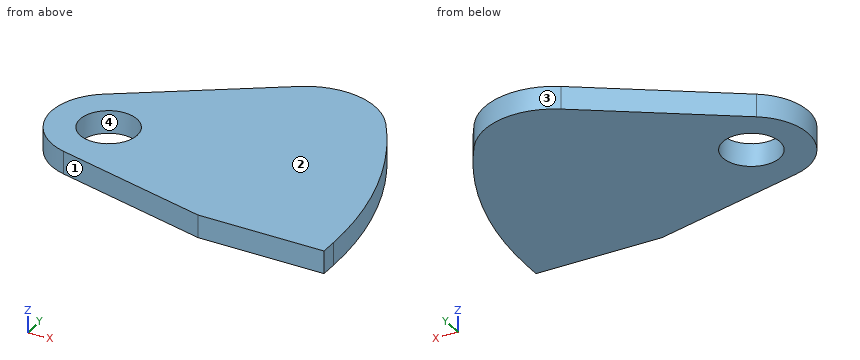
from build123d import *

# Parameters (mm, degrees)
SKETCH_1_R      = 5
EXTRUDE_1_DEPTH = 4


with BuildPart() as part:
    # Эскиз1 → Бобышка-Вытянуть1 (new body)
    with BuildSketch(Plane.XY):
        with BuildLine():
            Line((10.65, 0), (10.65, -3))
            Line((10.65, -3), (-11.397789553, -3))
            Line((-11.397789553, -3), (-38.677904755, 3.651503117))
            ThreePointArc((-38.677904755, 3.651503117), (-46.153775079, 11.6113462), (-41.890065439, 21.664630197))
            Line((-41.890065439, 21.664630197), (-17.065107401, 38.361673869))
            ThreePointArc((-17.065107401, 38.361673869), (-7.827814909, 40.223299164), (0.014835138, 34.999692982))
            ThreePointArc((0.014835138, 34.999692982), (7.932514626, 18.289923732), (10.65, 0))
        make_face()
        with Locations((-36.309076923, 13.366885492)):
            Circle(SKETCH_1_R, mode=Mode.SUBTRACT)
    extrude(amount=EXTRUDE_1_DEPTH)


solid = part.part
Read the model definition and answer for the solid it produces. Units are mm, in the model's axes. Face numbers are marked on the shaded views. Coordinates: 2 decimals unless noted, no trailing zeros. Order: outer loops, then holes, each group sorted by start corner. A loop starts at its lowest first (then second) coordinate and runs counter-clockwise, first axis right, second up. Notation, with made-up numbers: (41.25, 30.5) -> (47.25, 30.5) arc R22 cw to (47.25, 47.5) -> close; hole circle Ø2 at (82.25, -24.5). An arc over 180 degrees is marked (long way). Answer as a JSON object with one key per item and string values.
1) A cutting plane is placed at A-A, the plane y = 17.5. Determine the outline of the cut face in (x, z), plus the area to 3 significant figures.
Model answer:
{"outline": "(-45.41, 0) -> (-39.12, 0) -> (-39.12, 4) -> (-45.41, 4) -> close; (-33.5, 0) -> (8.17, 0) -> (8.17, 4) -> (-33.5, 4) -> close", "area": "192 mm²"}
2) A cutting plane is placed at B-B, the plane z = 1.7. Determine the outline of the cut face in (x, y).
Model answer:
{"outline": "(-41.89, 21.66) arc R10 ccw to (-38.68, 3.65) -> (-11.4, -3) -> (10.65, -3) -> (10.65, 0) arc R62.91 ccw to (0.01, 35) arc R12.3 ccw to (-17.07, 38.36) -> close; hole circle Ø10 at (-36.31, 13.37)"}
3) Each of these flat-tipped pins is pushed along its axis until it touches: pin 1 (1 mm diameter, centred on y = 27, z = 3, fed in from -X); pin 2 (8 mm diameter, centred on x = -23.5, y = 16, fed in from -Z); pin 3 (1 mm diameter, centred on x = -34.5, z = 3.5, fed in from +Y); pin 4 (1.5 mm diameter, centred on y = 9, z = 2, fed in from +X). Where does it stop, or does it pass through?
Model answer:
{"pin 1": "stops at x = -34.7", "pin 2": "stops at z = 0", "pin 3": "stops at y = 26.97", "pin 4": "stops at x = 10.11"}
4) The mould has two halves that part along X. Classify the marked faces 1, 2, 3 and 4: released by +X, released by -X, zero draft, split by the parting line, or undercut.
Model answer:
{"face 1": "released by -X", "face 2": "zero draft", "face 3": "split by the parting line", "face 4": "undercut"}
5) Consider line 1 along Y through (x, z) = (-35.5, 0.35); line 2 along X through (y, z) = (9.5, 1.4); line 3 along X through (y, z) = (15.5, 2.4). Determine where each line is inside the solid, lowest interval first. Write a range as from..to.
Model answer:
{"line 1": "y = 2.88..8.43, 18.3..25.96", "line 2": "x = -45.53..-39.48, -33.14..9.93", "line 3": "x = -46.08..-40.83, -31.79..8.71"}
6) A cutting plane is placed at D-D, the plane y = 25.5. Determine the outline of the cut face in (x, z).
Model answer:
{"outline": "(-36.19, 0) -> (5.25, 0) -> (5.25, 4) -> (-36.19, 4) -> close"}
7) A cutting plane is placed at C-C, the plane y = 9.5. Determine the outline of the cut face in (x, z).
Model answer:
{"outline": "(-45.53, 0) -> (-39.48, 0) -> (-39.48, 4) -> (-45.53, 4) -> close; (-33.14, 0) -> (9.93, 0) -> (9.93, 4) -> (-33.14, 4) -> close"}
